Geometry: final body of the model. Coordinates: model frame, mm. A direction names the side the tool comes from. Give positions to 0.01 mm unless a question says otherwise; leave off trailing zeros. Loops run counter-clockwise (first coordinate to the right, second up) from the corner with the lowest first, then second, coordinate; pieces in that order, holes last. Notation, with made-up numbers: (70.5, 61.5) - (102.5, 61.5) arc R32 ccw to (102.5, 88.5) - close; hole circle Ø5 at (62.25, 1.25). An arc over 180 degrees is marked (long way). Answer in a Markdown table with one row per item.
from build123d import *

# Parameters (mm, degrees)
SKETCH1_W           = 54
SKETCH1_H           = 50
BOSS_EXTRUDE1_DEPTH = 42
CHAMFER1_SIZE       = 10
SKETCH2_R           = 10
CUT_EXTRUDE1_DEPTH  = 51
SKETCH3_R           = 2.5
CUT_EXTRUDE2_DEPTH  = 15


with BuildPart() as part:
    # Sketch1 → Boss-Extrude1 (new body)
    with BuildSketch(Plane.XY):
        Rectangle(SKETCH1_W, SKETCH1_H)
    extrude(amount=BOSS_EXTRUDE1_DEPTH)

    # Chamfer1
    chamfer1_edges = [part.edges().sort_by_distance(p)[0] for p in [
        (27, 0, 0),
        (-27, 0, 0),
    ]]
    chamfer(chamfer1_edges, length=CHAMFER1_SIZE)

    # Sketch2 → Cut-Extrude1 (cut, through all)
    with BuildSketch(Plane(origin=(0, 25, 0), x_dir=(1, 0, 0), z_dir=(0, 1, 0))):
        with Locations((0, -21)):
            Circle(SKETCH2_R)
    extrude(amount=-CUT_EXTRUDE1_DEPTH, mode=Mode.SUBTRACT)

    # Sketch3 → Cut-Extrude2 (cut)
    with BuildSketch(Plane.XY.offset(42)):
        with Locations((-20, 20)):
            Circle(SKETCH3_R)
        with Locations((20, 20)):
            Circle(SKETCH3_R)
        with Locations((-20, -20)):
            Circle(SKETCH3_R)
        with Locations((20, -20)):
            Circle(SKETCH3_R)
    extrude(amount=-CUT_EXTRUDE2_DEPTH, mode=Mode.SUBTRACT)


solid = part.part
Q1. First-contact query: pin 1 (1.5 mm diameter, centred on x = -21, y = 20, fed in from +Z); pin 2 (4 mm diameter, centred on x = 20, y = -20, fed in from -Z); pin 3 (16 mm diameter, centred on x = 0, z = 21, fed in from +Y). Flat tips, straight axial feed; report the tip coordinate or a pass-through.
Check values:
| item | result |
|---|---|
| pin 1 | z = 27 |
| pin 2 | z = 1 |
| pin 3 | through |
Q2. Draft query along Y for faces 1 (the flat face through (6, -25, 30)), 2 (the flat face through (-22, 0, 5)), 3 (the cylindrical face through (17.5, -19.9, 34.6)). Return one class per face: pulls with the +Y half, pulls with the -Y half, needs draft (parallel to the pull), parting line crosses it, or undercut.
Check values:
| item | result |
|---|---|
| face 1 | pulls with the -Y half |
| face 2 | needs draft |
| face 3 | undercut |
Q3. Cut plane D-D (x = -20). Output: boundary loops of the cut face in (y, z), and give its area (3 significant figures).
Check values:
| item | result |
|---|---|
| outline | (-25, 3) - (25, 3) - (25, 42) - (22.5, 42) - (22.5, 27) - (17.5, 27) - (17.5, 42) - (-17.5, 42) - (-17.5, 27) - (-22.5, 27) - (-22.5, 42) - (-25, 42) - close |
| area | 1,800 mm² |
Q4. Cut plane C-C (y = -12). Output: boundary loops of the cut face in (x, z).
Check values:
| item | result |
|---|---|
| outline | (-27, 10) - (-17, 0) - (17, 0) - (27, 10) - (27, 42) - (-27, 42) - close; hole circle Ø20 at (0, 21) |
Q5. Cut plane A-A (x = 8). Output: boundary loops of the cut face in (y, z), and give its area (3 significant figures).
Check values:
| item | result |
|---|---|
| outline | (-25, 0) - (25, 0) - (25, 15) - (-25, 15) - close; (-25, 27) - (25, 27) - (25, 42) - (-25, 42) - close |
| area | 1,500 mm² |
Q6. Reachability of faces 4 (the flat face through (20, -20, 27)), 5 (the flat face through (6, 25, 30)) from +Z, -Z, +X, -X, +Y, -Y: full face, straight path, thin tool, end or side. Return the list, or none.
Check values:
| item | result |
|---|---|
| face 4 | +Z |
| face 5 | +Z, -Z, +X, -X, +Y |
Q7. Cut plane B-B (z = 13). Output: boundary loops of the cut face in (x, y), and give its area (3 significant figures).
Check values:
| item | result |
|---|---|
| outline | (-27, -25) - (-6, -25) - (-6, 25) - (-27, 25) - close; (6, -25) - (27, -25) - (27, 25) - (6, 25) - close |
| area | 2,100 mm² |
Q8. Material intervals for line 1 along Y through (x, z) = (20, 38.25); line 2 along X through (y, z) = (-18, 33); line 3 along X through (y, z) = (-7.5, 21), sorted ascending.
Check values:
| item | result |
|---|---|
| line 1 | -25 to -22.5, -17.5 to 17.5, 22.5 to 25 |
| line 2 | -27 to -21.5, -18.5 to 18.5, 21.5 to 27 |
| line 3 | -27 to -10, 10 to 27 |
